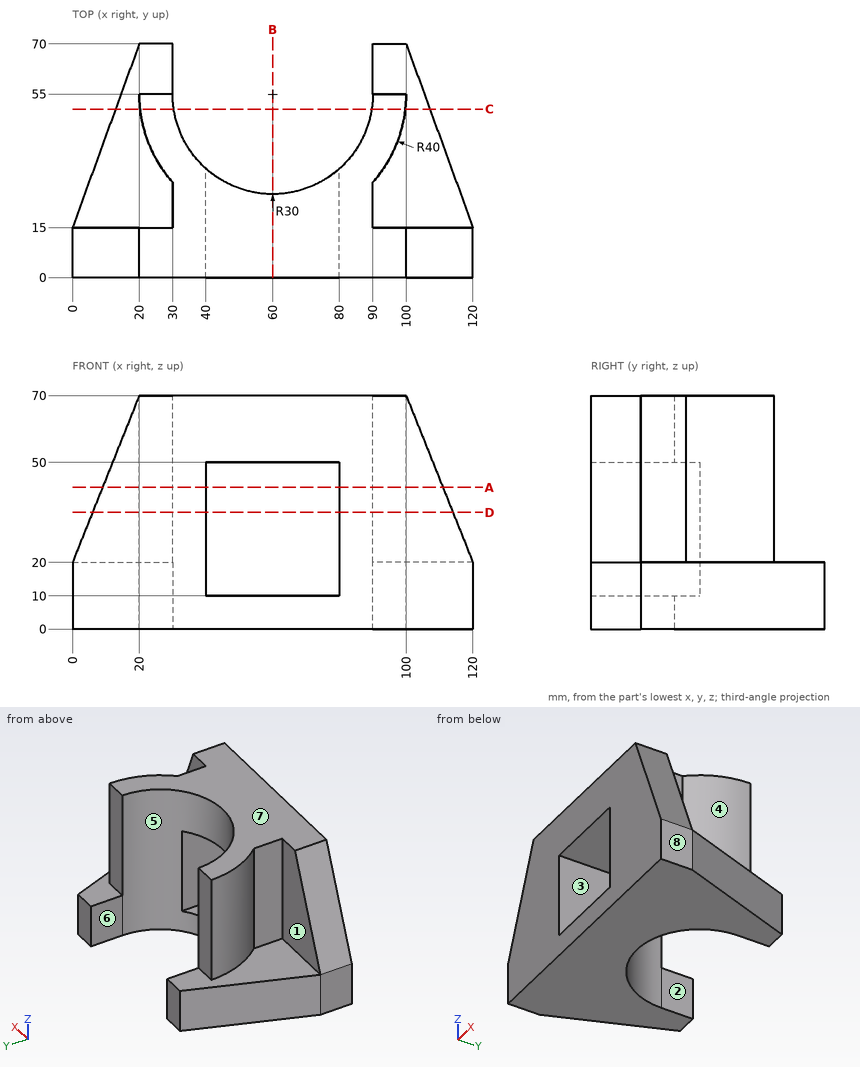
The drawing under review shows one solid part. Ordinate dimensions are in mm from its lowest x, y, z. A direction names the side the tool comes from. Give positions to 0.01 mm unless a question says otherwise; leave off trailing zeros. Write each loop counter-clockwise with the first axis right and the second up, starting at its lowest first coordinate (ties: lowest second). Pieces come first, ordered by that corner, then holes.
1. Add section C-C, the plane y = 50.5. Write out the cut boundary in (x, z).
2. Add section B-B, the plane x = 60. Write out the cut boundary in (y, z).
3. Tool access review of the marked faces 1, 2, 3 and 4: name each direction out of +Z, -Z, +X, -X, +Y, -Y from which nothing blocks a thin tool from reaching the whole face with its end or side.
4. For P1, Ø15, axis at y = 22, z = 54, coming from the +X side; P2, Ø11, axis at x = 97.5, z = 38.5, coming from the +Y side; P3, Ø3, axis at y = 52, z = 16, coming from the -X side, all flat-tipped, find the tip position at first contact; note any pin that passes through.
5. Wall thickness on L1, parallel to Z at x = 44.5, y = 20.5; L2, parallel to X at y = 21, z = 31.5; L3, parallel to X at y = 66, z = 19: over which ranges is each line inside the solid? List them lowest first.
6. Draft analysis for pull direction X (two halves, no side actions). For the marked faces 5, 6, 7 and 8, state which applies: +X half, -X half, draft (parallel to the pull), parting line (faces both ways), or undercut.
7. Add section D-D, the plane z = 35. Write out the cut boundary in (x, y), plus the area to 3 significant figures.
8. Add section A-A, the plane z = 42.5. Write out the cut boundary in (x, y).
Worked answers:
1. outline: (12.91, 0) - (30.34, 0) - (30.34, 70) - (20.25, 70) - (20.25, 20) - (12.91, 20) - close; (89.66, 0) - (107.09, 0) - (107.09, 20) - (99.75, 20) - (99.75, 70) - (89.66, 70) - close
2. outline: (0, 0) - (25, 0) - (25, 10) - (0, 10) - close; (0, 50) - (25, 50) - (25, 70) - (0, 70) - close
3. face 1: +Z, -X
3. face 2: +Z, -Z, +Y
3. face 3: +Y, -Y
3. face 4: +Z, +X
4. P1: stops at x = 107.48
4. P2: stops at y = 55
4. P3: stops at x = 12.91
5. L1: z = 0 to 10, 50 to 70
5. L2: x = 30 to 40, 80 to 90
5. L3: x = 18.55 to 30, 90 to 101.45
6. face 5: undercut
6. face 6: undercut
6. face 7: draft
6. face 8: +X half
7. outline: (6, 0) - (40, 0) - (40, 32.64) arc R30 cw to (30, 55) - (20, 55) arc R40 ccw to (30, 28.54) - (30, 15) - (6, 15) - close; (80, 0) - (114, 0) - (114, 15) - (90, 15) - (90, 28.54) arc R40 ccw to (100, 55) - (90, 55) arc R30 cw to (80, 32.64) - close
7. area: 1,870 mm2
8. outline: (9, 0) - (40, 0) - (40, 32.64) arc R30 cw to (30, 55) - (20, 55) arc R40 ccw to (30, 28.54) - (30, 15) - (9, 15) - close; (80, 0) - (111, 0) - (111, 15) - (90, 15) - (90, 28.54) arc R40 ccw to (100, 55) - (90, 55) arc R30 cw to (80, 32.64) - close
